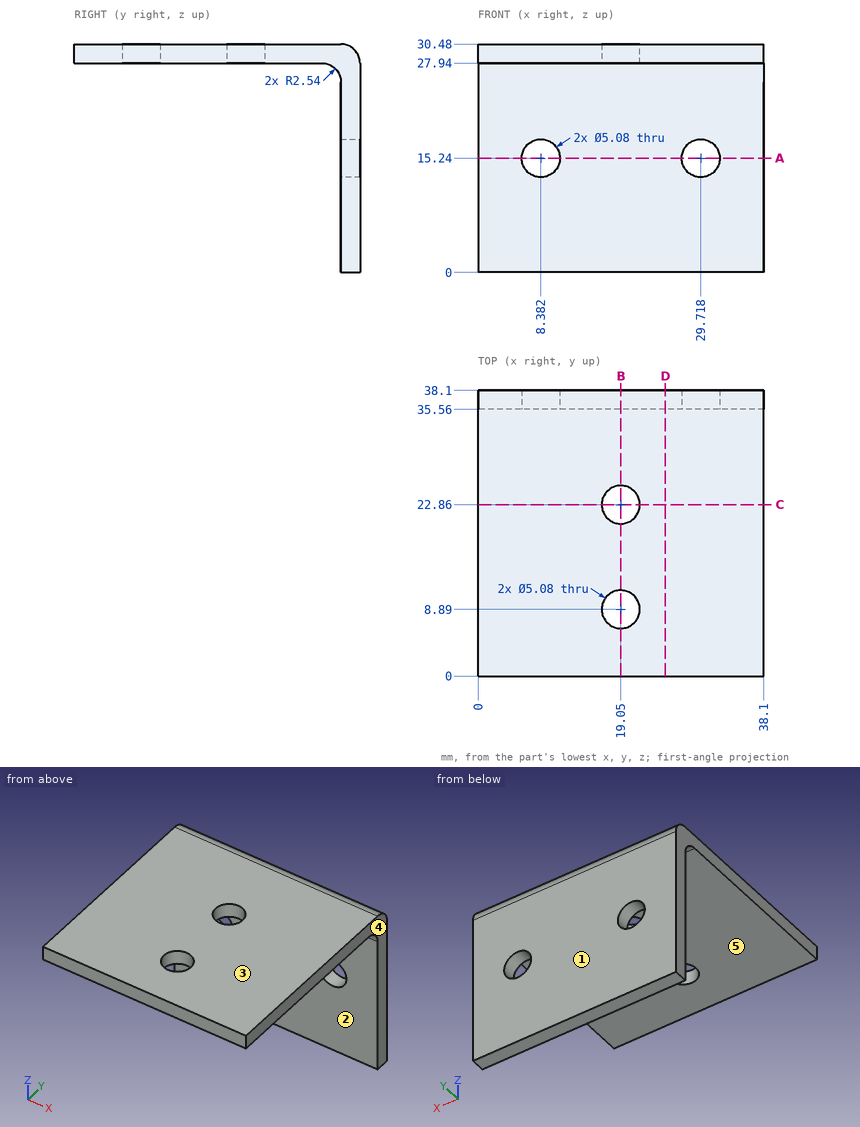
Geometry check sheet. Reference: drawing and pictorial views, mm from the part's lowest x, y, z. A direction names the side the tool comes from. Round coordinates to 2 decimals unless told otherwise and drop trailing zeros. Order: outer loops, then holes, each group sorted by start corner. A loop starts at its lowest first (then second) coordinate and runs counter-clockwise, first axis right, second up. Notation, with made-up numbers: M 60,-2 L 69,-2 A17 cw 69,29 Z; hole C -38,44 d1. An arc over 180 degrees is marked long. Write item = value, one per line.
Q1. Depth check by flat-ended pin: pin 1 Ø8 at (x, y) = (19.05, 22.86) entering from -Z; pin 2 Ø6 at (x, z) = (29.718, 15.24) entering from +Y. Enter the tip coordinate at first touch or a pass-through.
Answer block:
pin_1 = 27.94
pin_2 = 38.1
Q2. Release check for a two-part mould opening along Y. For the marked faces 1, 2 and 3 record: released by +Y, released by -Y, zero draft, split by the parting line, or undercut.
Answer block:
face_1 = released by +Y
face_2 = released by -Y
face_3 = zero draft
Q3. Section check D-D (x = 25). Enter the section's corners in (y, z), plus the area to 3 significant figures.
Answer block:
outline = M 0,27.94 L 33.02,27.94 A2.54 cw 35.56,25.4 L 35.56,0 L 38.1,0 L 38.1,27.94 A2.54 ccw 35.56,30.48 L 0,30.48 Z
area = 168 mm^2
Q4. Scan lines: line 1 (Y direction, x = 19.05, z = 29.25); line 2 (Y direction, x = 19, z = 29); line 3 (Z direction, x = 36, y = 22). Record each from-to range of solid material in increasing order.
Answer block:
line_1 = 0 to 6.35, 11.43 to 20.32, 25.4 to 37.74
line_2 = 0 to 6.35, 11.43 to 20.32, 25.4 to 37.87
line_3 = 27.94 to 30.48
Q5. Set-up check for the marked faces 4 and 5: record each of +Z, -Z, +X, -X, +Y, -Y from which the full face is reachable in a straight line by a thin tool's end or side.
Answer block:
face_4 = +Z, -Z, +X, +Y, -Y
face_5 = -Z, +X, -X, -Y
Q6. Section check A-A (z = 15.24). Enter the section's corners in (x, y), plus the area to 3 significant figures.
Answer block:
outline = M 0,35.56 L 5.84,35.56 L 5.84,38.1 L 0,38.1 Z; M 10.92,35.56 L 27.18,35.56 L 27.18,38.1 L 10.92,38.1 Z; M 32.26,35.56 L 38.1,35.56 L 38.1,38.1 L 32.26,38.1 Z
area = 71.0 mm^2
Q7. Section check C-C (y = 22.86). Enter the section's corners in (x, z), plus the area to 3 significant figures.
Answer block:
outline = M 0,27.94 L 16.51,27.94 L 16.51,30.48 L 0,30.48 Z; M 21.59,27.94 L 38.1,27.94 L 38.1,30.48 L 21.59,30.48 Z
area = 83.9 mm^2
Q8. Section check B-B (x = 19.05). Enter the section's corners in (y, z).
Answer block:
outline = M 0,27.94 L 6.35,27.94 L 6.35,30.48 L 0,30.48 Z; M 11.43,27.94 L 20.32,27.94 L 20.32,30.48 L 11.43,30.48 Z; M 25.4,27.94 L 33.02,27.94 A2.54 cw 35.56,25.4 L 35.56,0 L 38.1,0 L 38.1,27.94 A2.54 ccw 35.56,30.48 L 25.4,30.48 Z
